Print and shaded views of the part. All mm, measured from the part's lowest x, y and z. A direction names the side the tool comes from. Round coordinates to 2 decimals unless told otherwise and drop trailing zeros. Write each loop counter-clockwise with the first axis right and the second up, starting at its lowest first coordinate (ties: lowest second). Pieces come first, ordered by that corner, then holes. Notation, with made-up numbers: M -18.75,40 L -2.75,40 A24 ccw -2.75,57 Z; hole C -10,52.5 d4. An arc over 180 degrees is marked long. Write item = value, one per line.
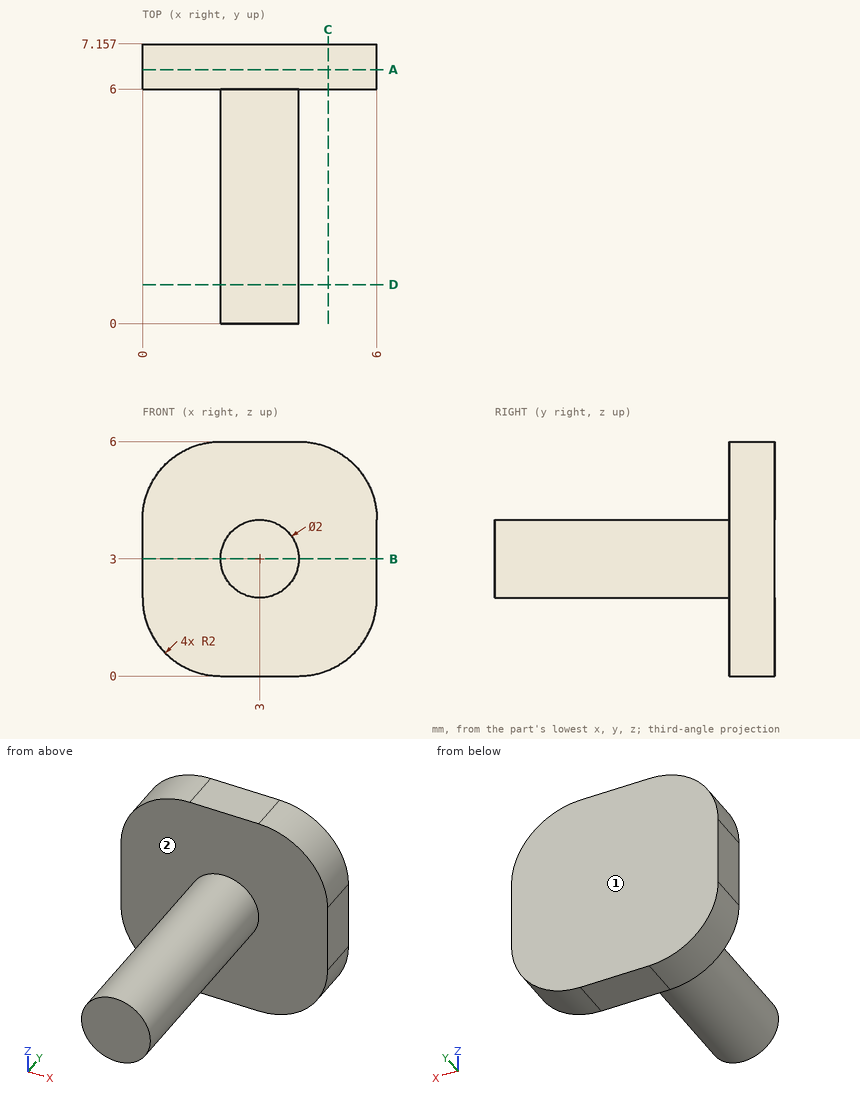
1. Band-saw the part on A-A (y = 6.5). List the corners of the cut face in (x, z).
Responses:
outline = M 0,2 A2 ccw 2,0 L 4,0 A2 ccw 6,2 L 6,4 A2 ccw 4,6 L 2,6 A2 ccw 0,4 Z
2. Band-saw the part on D-D (y = 1). List the corners of the cut face in (x, z), plus the area to 3 significant figures.
Responses:
outline = C 3,3 d2
area = 3.14 mm²
3. Probe probe 1 along Y at (x, z) = (0.5, 4.25); probe 2 along X at (y, z) = (0.5, 3); probe 3 along Z at (x, y) = (2.5, 3.75). List the from-to ranges inside material, lowest first.
Responses:
probe_1 = 6 to 7.16
probe_2 = 2 to 4
probe_3 = 2.13 to 3.87
4. Flat gauge pins, fed straight in: pin 1 (1 mm diameter, centred on x = 3, y = 6, fed in from -Z); pin 2 (1 mm diameter, centred on x = 2, y = 2, fed in from +Z). Where does each tip first touch, or does it go through?
Responses:
pin_1 = 0
pin_2 = 3.87
5. Band-saw the part on C-C (x = 4.75). List the corners of the cut face in (y, z).
Responses:
outline = M 6,0.15 L 7.16,0.15 L 7.16,5.85 L 6,5.85 Z
6. Tool access for the marked faces 1 and 2: list every direction of +Z, -Z, +X, -X, +Y, -Y with a clear straight run to the whole face (end or side of a thin tool).
Responses:
face_1 = +Z, -Z, +X, -X, +Y
face_2 = -Y
7. Band-saw the part on B-B (z = 3). List the corners of the cut face in (x, y), plus the area to 3 significant figures.
Responses:
outline = M 0,6 L 2,6 L 2,0 L 4,0 L 4,6 L 6,6 L 6,7.16 L 0,7.16 Z
area = 18.9 mm²
